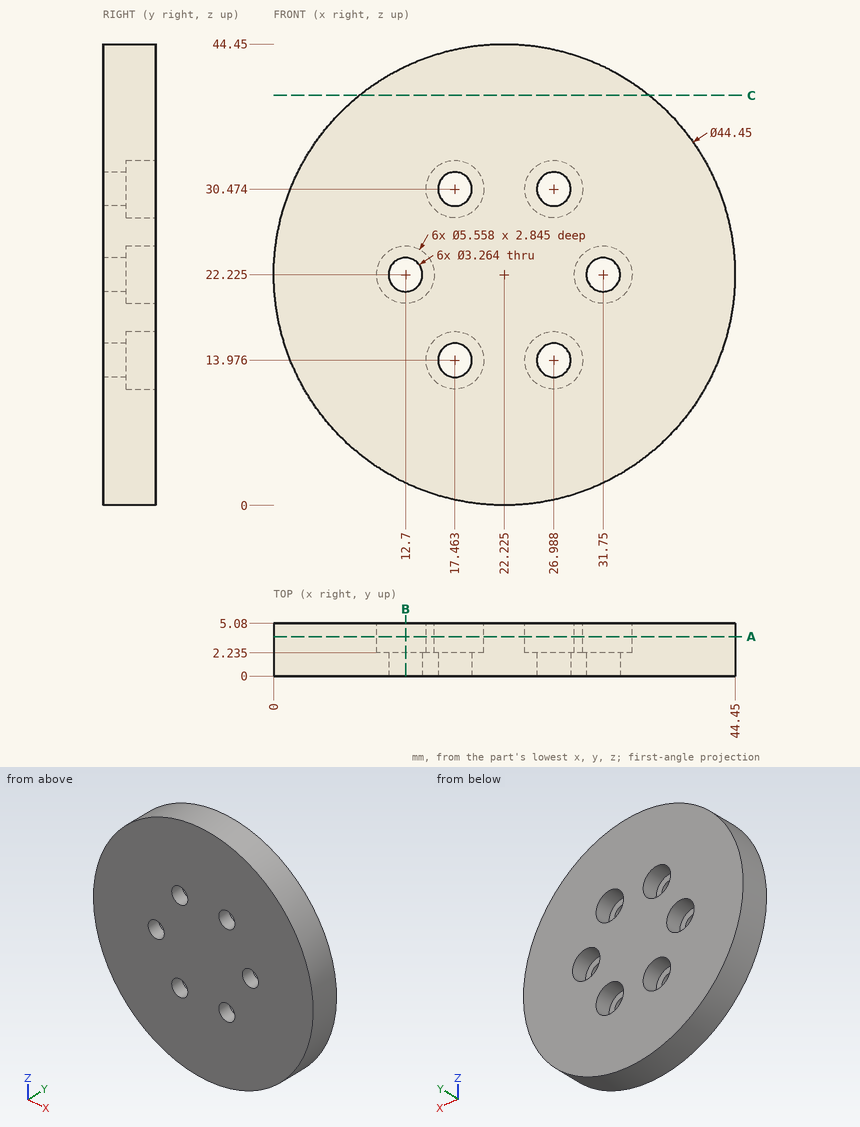
The figure shows three views and two pictorial views of one solid part (mm, origin at its lowest corner). Answer the questions. Coordinates: 2 decimals unless noted, no trailing zeros. Write each loop counter-clockwise with the first axis right and the second up, starting at its lowest first coordinate (ties: lowest second). Pieces come first, ordered by that corner, then holes. Notation, with made-up numbers: (1.25, 9) -> (44.25, 9) arc R22 ccw to (44.25, 25) -> close; hole circle Ø1 at (-8, 64). An arc over 180 degrees is marked (long way). Return JSON: item names as keys, results as strings.
1. Find the intervals of material crossed by line 1 along Z through (x, y) = (27.5, 4) (1 decimal); line 2 along Z through (x, y) = (19, 4.7) (1 decimal); line 3 along X through (y, z) = (1.1, 31) (1 decimal), in increasing order. Write a range as from..to.
Found:
{"line 1": "0.6..11.2, 16.7..27.7, 33.2..43.8", "line 2": "0.2..11.7, 16.3..28.2, 32.8..44.2", "line 3": "1.8..15.9, 19..25.4, 28.5..42.6"}
2. A cutting plane is placed at C-C (z = 39.5). Determine the outline of the cut face in (x, y), and give its area (3 significant figures).
Found:
{"outline": "(8.24, 0) -> (36.21, 0) -> (36.21, 5.08) -> (8.24, 5.08) -> close", "area": "142 mm2"}
3. Each of these flat-tipped pins is pushed along its axis until it touches: P1, Ø1, axis at y = 1.5, z = 14.5, coming from the -X side; P2, Ø1.7, axis at x = 17.5, z = 15, coming from the +Y side (1 decimal); P3, Ø2.5, axis at x = 31.75, z = 22.225, coming from the -Y side; P4, Ø1.5, axis at y = 4, z = 11.5, coming from the -X side (1 decimal). Where does it stop, or does it pass through?
Found:
{"P1": "x = 1.21", "P2": "y = 2.2", "P3": "through", "P4": "x = 2.4"}
4. A cutting plane is placed at B-B (x = 12.7). Determine the outline of the cut face in (y, z) (1 decimal).
Found:
{"outline": "(0, 2.1) -> (5.1, 2.1) -> (5.1, 19.4) -> (2.2, 19.4) -> (2.2, 20.6) -> (0, 20.6) -> close; (0, 23.9) -> (2.2, 23.9) -> (2.2, 25) -> (5.1, 25) -> (5.1, 42.3) -> (0, 42.3) -> close"}
5. A cutting plane is placed at A-A (y = 3.8). Give the number of separate pieces and of enclosed holes in the cut face, and give its area (3 significant figures).
Found:
{"separate pieces": "1", "enclosed holes": "6", "area": "1,410 mm2"}
